Print and shaded views of the part. All mm, measured from the part's lowest x, y and z. A direction names the side the tool comes from. Round coordinates to 2 decimals unless told otherwise and drop trailing zeros. Write each loop counter-clockwise with the first axis right and the second up, starting at its lowest first coordinate (ties: lowest second). Pieces come first, ordered by that corner, then holes. Notation, with made-up numbers: (55.25, 37.5) -> (104.25, 37.5) arc R12 cw to (104.25, 42.5) -> close; hole circle Ø10 at (42.25, 58.25). An arc over 180 degrees is marked (long way). Return JSON: item names as keys, results as strings. Group by question number.
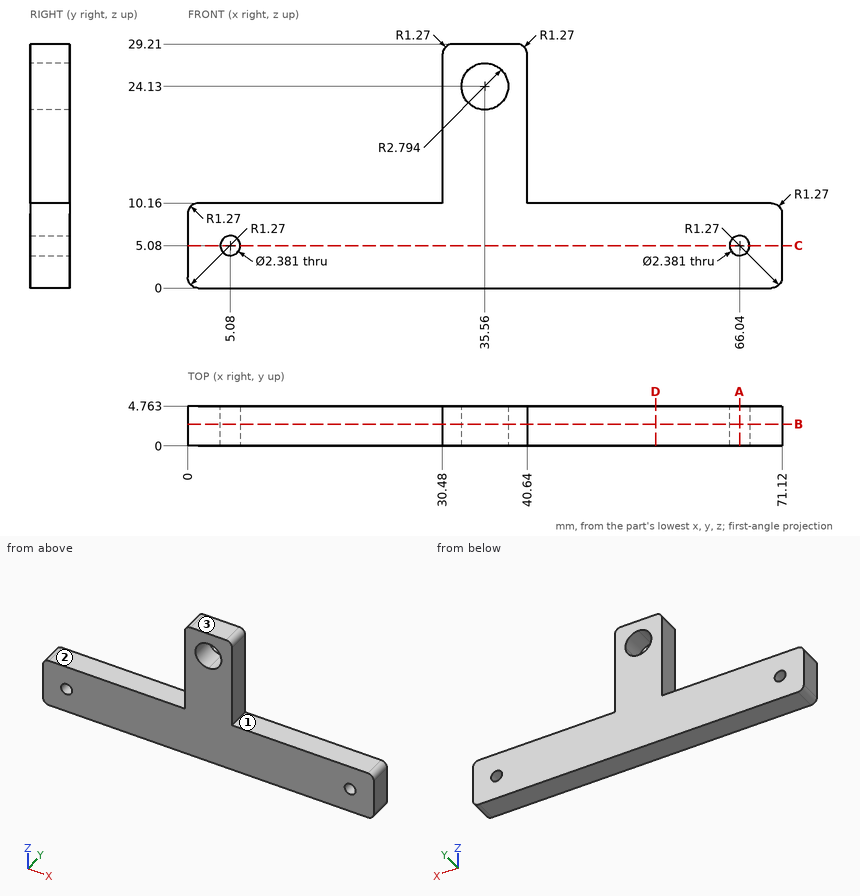
Item 1: Wall check: L1, parallel to Z at x = 66.04, y = 3.6; L2, parallel to Z at x = 14, y = 2.1; L3, parallel to X at y = 3.3, z = 4.5. Give the ranges that are in metal, low to high.
Item 2: Cut at A-A (x = 66.04). Write the cut outline in (y, z).
Item 3: Cut at B-B (y = 2.6). State how many separate pieces and enclosed holes the cut face has.
Item 4: Which spindle directions (+Z, -Z, +X, -X, +Y, -Y) get a long thin tool onto all of the face, cutting with end or side? Do the marked faces 1, 2 and 3. Say none if no direction does.
Item 5: Flat gauge pins, fed straight in: P1, Ø5, axis at x = 41, z = 17.5, coming from the -Y side; P2, Ø2.5, axis at y = 1.5, z = 18, coming from the +X side; P3, Ø1.5, axis at y = 0.5, z = 16, coming from the -X side; P4, Ø2, axis at x = 24.5, y = 4.5, coming from the +Z side. Where does each tip first touch, or does it go through?
Item 6: Cut at D-D (x = 56). Write the cut outline in (y, z).
Item 7: Cut at C-C (z = 5.08). Write the cut outline in (x, y).
Checks:
{
 "1": {"L1": "z = 0 to 3.89, 6.27 to 10.16", "L2": "z = 0 to 10.16", "L3": "x = 0 to 4.04, 6.12 to 65, 67.08 to 71.12"},
 "2": {"outline": "(0, 0) -> (4.76, 0) -> (4.76, 3.89) -> (0, 3.89) -> close; (0, 6.27) -> (4.76, 6.27) -> (4.76, 10.16) -> (0, 10.16) -> close"},
 "3": {"separate pieces": "1", "enclosed holes": "3"},
 "4": {"face 1": "+Z, +X, +Y, -Y", "face 2": "+Z, -X, +Y, -Y", "face 3": "+Z, +X, -X, +Y, -Y"},
 "5": {"P1": "stops at y = 0", "P2": "stops at x = 40.64", "P3": "stops at x = 30.48", "P4": "stops at z = 10.16"},
 "6": {"outline": "(0, 0) -> (4.76, 0) -> (4.76, 10.16) -> (0, 10.16) -> close"},
 "7": {"outline": "(0, 0) -> (3.89, 0) -> (3.89, 4.76) -> (0, 4.76) -> close; (6.27, 0) -> (64.85, 0) -> (64.85, 4.76) -> (6.27, 4.76) -> close; (67.23, 0) -> (71.12, 0) -> (71.12, 4.76) -> (67.23, 4.76) -> close"}
}
